```python
from build123d import *

# Parameters (mm, degrees)
F1_DEPTH = 266.7
F3_DEPTH = 76.2


with BuildPart() as f1:
    # F0 (on Front) → F1 (new body, symmetric)
    with BuildSketch(Plane.XZ):
        Polygon((-38.1, -38.1), (38.1, -38.1), (38.1, -31.75), (-31.75, -31.75), (-31.75, 38.1), (-38.1, 38.1), align=None)
    extrude(amount=F1_DEPTH, both=True)

    # F2 (on face) → F3 (cut)
    with BuildSketch(Plane(origin=(-38.1, 0, 0), x_dir=(0, -1, 0), z_dir=(-1, 0, 0))):
        Polygon((-266.7, 38.1), (-266.7, -38.1), (-190.5, 38.1), align=None)
    extrude(amount=-F3_DEPTH, mode=Mode.SUBTRACT)


solid = f1.part
```
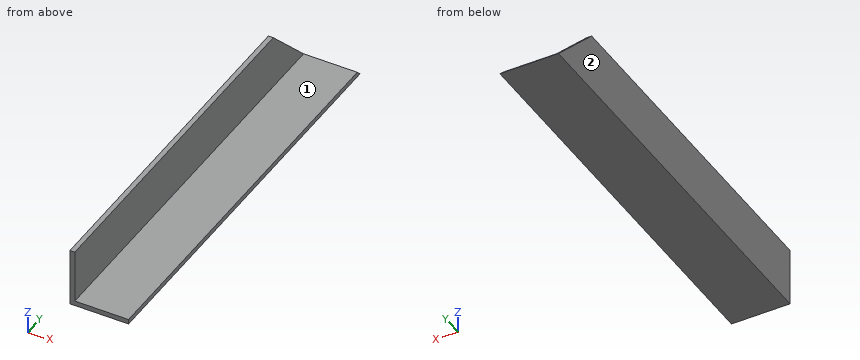
Geometry: final body of the model. Coordinates: model frame, mm. Face numbers are marked on the shaded views. A direction names the side the tool comes from. Round coordinates to 2 decimals unless told otherwise and drop trailing zeros. Order: outer loops, then holes, each group sorted by start corner. A loop starts at its lowest first (then second) coordinate and runs counter-clockwise, first axis right, second up. Notation, with made-up numbers: (-25, 69.5) -> (31, 69.5) arc R26 ccw to (31, 104.5) -> close; hole circle Ø10 at (29.25, -6.5). An arc over 180 degrees is marked (long way). Use one line per item in the form item = value. Start each with the question number.
1. Reachability of the marked faces 1 and 2 from +Z, -Z, +X, -X, +Y, -Y: full face, straight path, thin tool, end or side. Return the list, or none.
2. Cut plane D-D (y = 155.5). Return the cut outline in (x, z), then the cut area to 3 significant figures.
3. Cut plane A-A (y = 223). Return the cut outline in (x, z), then the cut area to 3 significant figures.
4. Line query: probe 1 along Z at (x, y) = (-19.5, -226.5); probe 2 along Y at (x, z) = (-2, -34.5). Output: solid intervals per line, ascending.
5. Cut plane B-B (z = -20). Return the cut outline in (x, y).
6. Cut plane C-C (x = 1). Return the cut outline in (y, z), then the cut area to 3 significant figures.
7. Pin query (flat end, axial travel): pin 1 Ø4 at (x, y) = (-19.5, -139.5) entering from +Z; pin 2 Ø12 at (x, z) = (-8.5, -24.5) entering from +Y; pin 3 Ø12 at (x, z) = (-26.5, -16.5) entering from +Y; pin 4 Ø6 at (y, z) = (-81, 1.5) entering from +X. Return the tip coordinate at first contact, or that it passes through.
Solution:
q1.face_1 = +Z, +X, +Y, -Y
q1.face_2 = +Z, -Z, -X, +Y, -Y
q2.outline = (-38.1, -38.1) -> (38.1, -38.1) -> (38.1, -31.75) -> (-31.75, -31.75) -> (-31.75, 38.1) -> (-38.1, 38.1) -> close
q2.area = 927 mm^2
q3.outline = (-38.1, -38.1) -> (38.1, -38.1) -> (38.1, -31.75) -> (-31.75, -31.75) -> (-31.75, 5.6) -> (-38.1, 5.6) -> close
q3.area = 721 mm^2
q4.probe_1 = -38.1 to -31.75
q4.probe_2 = -266.7 to 263.1
q5.outline = (-38.1, -266.7) -> (-31.75, -266.7) -> (-31.75, 248.6) -> (-38.1, 248.6) -> close
q6.outline = (-266.7, -38.1) -> (266.7, -38.1) -> (260.35, -31.75) -> (-266.7, -31.75) -> close
q6.area = 3,370 mm^2
q7.pin_1 = -31.75
q7.pin_2 = through
q7.pin_3 = 248
q7.pin_4 = -31.75
